from build123d import *

# Parameters (mm, degrees)
SKETCH1_W           = 66
SKETCH1_H           = 12
SKETCH1_R           = 2.98
BOSS_EXTRUDE1_DEPTH = 20
FILLET2_R           = 6


with BuildPart() as part:
    # Sketch1 → Boss-Extrude1 (new, symmetric)
    with BuildSketch(Plane.XY):
        with Locations((27, 0)):
            Rectangle(SKETCH1_W, SKETCH1_H)
        Circle(SKETCH1_R, mode=Mode.SUBTRACT)
    extrude(amount=BOSS_EXTRUDE1_DEPTH, both=True)

    # Fillet2
    fillet2_edges = [part.edges().sort_by_distance(p)[0] for p in [
        (60, -6, 0),
        (60, 6, 0),
        (-6, -6, 0),
        (-6, 6, 0),
    ]]
    fillet(fillet2_edges, radius=FILLET2_R - 0.0001)  # a hair under: the kernel refuses the full size


solid = part.part
The listing builds one solid part. Answer for the finished solid, in the listing's coordinates (mm). Round coordinates to 2 decimals unless told otherwise and drop trailing zeros. Order: outer loops, then holes, each group sorted by start corner. A loop starts at its lowest first (then second) coordinate and runs counter-clockwise, first axis right, second up. Notation, with made-up numbers: (74.5, 24.25) -> (85.5, 24.25) arc R19 cw to (85.5, 33.25) -> close; hole circle Ø3 at (-15, 58.25). An arc over 180 degrees is marked (long way). Put each result on its own line as item: value.
Q1. Each of these flat-tipped pins is pushed along its axis until it touches: P1, Ø2, axis at y = 3, z = 14, coming from the +X side; P2, Ø3, axis at y = -0.5, z = 10, coming from the +X side; P3, Ø3, axis at y = -4, z = -1, coming from the -X side; P4, Ø4, axis at y = 2.5, z = 5, coming from the -X side. Where does it stop, or does it pass through?
Results list:
P1: x = 59.66
P2: x = 60
P3: x = -5.45
P4: x = -5.98
Q2. Section C-C, the plane y = 5 is taken. Write down the section's boundary in (x, z).
Results list:
outline: (-3.32, -20) -> (57.32, -20) -> (57.32, 20) -> (-3.32, 20) -> close
Q3. Consider line 1 along Y through (x, z) = (0, -5.5); line 2 along Y through (x, z) = (2, -11.5); line 3 along X through (y, z) = (1.5, -4.5). Determine where each line is inside the solid, lowest interval first.
Results list:
line 1: -6 to -2.98, 2.98 to 6
line 2: -6 to -2.21, 2.21 to 6
line 3: -5.81 to -2.57, 2.57 to 59.81
Q4. Section A-A, the plane y = 0.75 is taken. Write down the section's boundary in (x, z).
Results list:
outline: (-5.95, -20) -> (-2.88, -20) -> (-2.88, 20) -> (-5.95, 20) -> close; (2.88, -20) -> (59.95, -20) -> (59.95, 20) -> (2.88, 20) -> close
Q5. Section D-D, the plane y = -4 is taken. Write down the section's boundary in (x, z).
Results list:
outline: (-4.47, -20) -> (58.47, -20) -> (58.47, 20) -> (-4.47, 20) -> close
Q6. Determine the mould class of faces 1 (the cylindrical face through (-0.388, 2.955, -0.28)), 2 (the flat face through (27, 6, 0)), 3 (the cylindrical face through (-4.289, 4.196, -0.28)) for opening direction X: pulls with the +X half, pulls with the -X half, needs draft (parallel to the pull), parting line crosses it, or undercut.
Results list:
face 1: undercut
face 2: needs draft
face 3: pulls with the -X half
